Could you check a few things on this model? Use its own coordinates, in mm. A direction names the side the tool comes from. Round coordinates to 2 decimals unless told otherwise and drop trailing zeros. Write each loop counter-clockwise with the first axis right and the second up, starting at its lowest first coordinate (ties: lowest second). Pieces come first, ordered by that corner, then holes. Notation, with made-up numbers: (-32, 29.5) - (21, 29.5) arc R19 ccw to (21, 36.5) - close; hole circle Ø3 at (-17.75, 49.5). An arc over 180 degrees is marked (long way). Write each question's results on one line, items separated by ' | '. Start each with the question number.
(1) On a 3-axis mill with a long thin cutter (end or side, diameter ignored), from which of +Z, -Z, +X, -X, +Y, -Y can I reach the whole of each face in a straight line? I mean faces 1 (the flat face through (15, 9, 0)), 2 (the flat face through (0, 6, 0)). Say none if no direction works.
(2) Imagine slicing it at D-D on z = 4.5. Write out the boundary of the cut face in (x, y), then the cut area to 3 significant figures.
(3) Thinking about a two-plate mould opening in Z: for faces 3 (the flat face through (0, 9, -1.75)), 4 (the flat face through (0, 10, 2)), 5 (the flat face through (0, 8, 8)), 6 (the flat face through (0, 8, -8)), which applies, +Z half, -Z half, draft (parallel to the pull), parting line (faces both ways), or undercut?
(4) Imagine slicing it at B-B on x = -9. Write out the boundary of the cut face in (y, z).
(5) Imagine slicing it at C-C on z = 0.75. Write out the boundary of the cut face in (x, y), then the cut area to 3 significant figures.
(6) For P1, Ø1, axis at y = 8, z = 6, coming from the -X side; P2, Ø1.8, axis at x = -1, z = 0, coming from the +Y side; P3, Ø1.5, axis at y = 7, z = 3.5, coming from the +X side, each with a flat end and sliding along its axis, tell me the tip position at first contact or that it passes through.
(7) Please list where these lines run through material, in increasing order: line 1 (Z direction, x = -8.5, y = 7.05); line 2 (X direction, y = 7.65, z = 1.5); line 3 (Y direction, x = 4.5, z = 0.25). Write a range as [from, to].
(8) Imagine slicing it at A-A on y = 8.05. Write out the boundary of the cut face in (x, z), then the cut area to 3 significant figures.
Autodesk Inventor part; units mm, degrees
ref_plane "YZ Plane" through (0, 0, 0) normal (1, 0, 0) x (0, 1, 0)
ref_plane "XZ Plane" through (0, 0, 0) normal (0, 1, 0) x (-1, 0, 0)
ref_plane "XY Plane" through (0, 0, 0) normal (0, 0, 1) x (1, 0, 0)
sketch "Sketch1" plane through (0, 0, 0) normal (0, 1, 0) x (-1, 0, 0)
  circle A0 centre (0, 0) radius 25
  dimension "d2" = 50
extrude "Extrusion1" add sketch "Sketch1" along normal blind 10
sketch "Sketch2" plane through (0, 10, 0) normal (0, 1, 0) x (1, 0, 0)
  line L0 (-15, -1.75) -> (15, -1.75)
  line L1 (15, -1.75) -> (15, 1.75)
  line L2 (15, 1.75) -> (-15, 1.75)
  line L3 (-15, 1.75) -> (-15, -1.75)
  circle A0 centre (0, 0) radius 25
  point P0 (-25, 0)
  point P1 (0, 25)
  dimension "d5" = 30
  dimension "d6" = 3.5
  dimension "d7" = 23.25
  dimension "d8" = 10
extrude "Extrusion2" cut sketch "Sketch2" against normal blind 3 contours L3 L2 L1 L0
sketch "Sketch3" plane through (0, 10, 0) normal (0, 1, 0) x (1, 0, 0)
  line L0 (-38.0663, 8) -> (91.0616, 8)
  line L1 (-15, 1.75) -> (15, 1.75)
  arc A0 (91.0616, 8) -> (-38.0663, 8) centre (26.4976, -23.1626) ccw
  circle A1 centre (0, 0) radius 25 construction
  line L2 (-25, 0) -> (81.9095, 0) construction
  line L3 (-38.0663, -8) -> (91.0616, -8)
  arc A2 (-38.0663, -8) -> (91.0616, -8) centre (26.4976, 23.1626) ccw
  point P0 (24.7878, -3.25)
  dimension "d11" = 6.25
extrude "Extrusion3" cut sketch "Sketch3" against normal blind 10
sketch "Sketch4" plane through (0, 0, 0) normal (0, -1, 0) x (1, 0, 0)
  line L0 (-23.6854, -8) -> (23.6854, -8)
  arc A0 (23.6854, -8) -> (23.6854, 8) centre (0, 0) ccw
  line L1 (23.6854, 8) -> (-23.6854, 8)
  arc A1 (-23.6854, 8) -> (-23.6854, -8) centre (0, 0) ccw
extrude "Extrusion4" cut sketch "Sketch4" against normal blind 6
properties part number "planetstand"
Response:
1) face 1: +Y | face 2: +Z, -Z, +X, -X, -Y
2) outline: (-24.59, 6) - (24.59, 6) - (24.59, 10) - (-24.59, 10) - close | area: 197 mm²
3) face 3: undercut | face 4: draft | face 5: +Z half | face 6: -Z half
4) outline: (6, -8) - (10, -8) - (10, -1.75) - (7, -1.75) - (7, 1.75) - (10, 1.75) - (10, 8) - (6, 8) - close
5) outline: (-24.99, 6) - (24.99, 6) - (24.99, 10) - (15, 10) - (15, 7) - (-15, 7) - (-15, 10) - (-24.99, 10) - close | area: 110 mm²
6) P1: x = -24.39 | P2: y = 7 | P3: x = 24.85
7) line 1: [-8, -1.75], [1.75, 8] | line 2: [-24.95, -15], [15, 24.95] | line 3: [6, 7]
8) outline: (-23.69, -8) - (23.69, -8) arc R25 ccw to (23.69, 8) - (-23.69, 8) arc R25 ccw to start; hole (-15, -1.75) - (15, -1.75) - (15, 1.75) - (-15, 1.75) - close | area: 681 mm²
